Read the model definition and answer for the solid it produces. Units are mm, in the model's axes. A direction names the side the tool comes from. Round coordinates to 2 decimals unless told otherwise and drop trailing zeros. Loops run counter-clockwise (first coordinate to the right, second up) from the corner with the lowest first, then second, coordinate; pieces in that order, holes last. Notation, with made-up numbers: (45, 20) -> (59, 20) arc R11 cw to (59, 40) -> close; hole circle Ø7 at (49.5, 68). An arc over 180 degrees is marked (long way). Put each result on its own line as item: value.
from build123d import *

# Parameters (mm, degrees)
SKETCH1_R           = 2
BOSS_EXTRUDE1_DEPTH = 5
BOSS_EXTRUDE2_DEPTH = 1.5


with BuildPart() as part:
    # Sketch1 → Boss-Extrude1 (new body)
    with BuildSketch(Plane(origin=(0, 0, 0), x_dir=(1, 0, 0), z_dir=(0, 1, 0))):
        with Locations(Location((0, 0, 0), (0, 0, 270))):
            Circle(SKETCH1_R)
    extrude(amount=BOSS_EXTRUDE1_DEPTH)

    # Sketch2 → Boss-Extrude2 (add)
    with BuildSketch(Plane(origin=(0, 5, 0), x_dir=(1, 0, 0), z_dir=(0, 1, 0))):
        Polygon((4.828427125, 2), (2, 4.828427125), (-2, 4.828427125), (-4.828427125, 2), (-4.828427125, -2), (-2, -4.828427125), (2, -4.828427125), (4.828427125, -2), align=None)
    extrude(amount=BOSS_EXTRUDE2_DEPTH)


solid = part.part
Item 1: Find the intervals of material crossed by line 1 along Y through (x, z) = (-1.5, 4.25); line 2 along Z through (x, y) = (1.5, 4.5), in increasing order.
Derived:
line 1: y = 5 to 6.5
line 2: z = -1.32 to 1.32
Item 2: A flat-ended cylindrical pin translates along its axis: pin 1 Ø2 at (x, z) = (0, -2.5) entering from -Y. Find the tip coordinate at first contact, or state that the pin passes through.
Derived:
pin 1: stops at y = 0
Item 3: Which of the six approach directions +Z, -Z, +X, -X, +Y, -Y give full straight-line access (tool end or side, diameter ignored) to faces 1 (the flat face through (3.394, 5.74, 3.434)), 2 (the flat face through (-0.1, 5, -2.2))?
Derived:
face 1: +Z, +X, +Y, -Y
face 2: -Y
Item 4: The part is cut by section C-C (y = 4.5). Determine the outline of the cut face in (x, z).
Derived:
outline: circle Ø4 at (0, 0)
Item 5: The part is cut by section D-D (x = 3.5). Determine the outline of the cut face in (y, z), then the cut area to 3 significant figures.
Derived:
outline: (5, -3.33) -> (6.5, -3.33) -> (6.5, 3.33) -> (5, 3.33) -> close
area: 9.99 mm^2
Item 6: The part is cut by section A-A (x = 0). Determine the outline of the cut face in (y, z), then the cut area to 3 significant figures.
Derived:
outline: (0, -2) -> (5, -2) -> (5, -4.83) -> (6.5, -4.83) -> (6.5, 4.83) -> (5, 4.83) -> (5, 2) -> (0, 2) -> close
area: 34.5 mm^2
Item 7: The part is cut by section B-B (z = 0). Determine the outline of the cut face in (x, y), then the cut area to 3 significant figures.
Derived:
outline: (-4.83, 5) -> (-2, 5) -> (-2, 0) -> (2, 0) -> (2, 5) -> (4.83, 5) -> (4.83, 6.5) -> (-4.83, 6.5) -> close
area: 34.5 mm^2
